from build123d import *

# Parameters (mm, degrees)
PAD050_DEPTH = 5
SKETCH054_R  = 10
PAD051_DEPTH = 5
SKETCH055_R  = 2.2
HOLE_DEPTH   = 25
SKETCH056_R  = 3
POCKET_DEPTH = 10.001


with BuildPart() as part:
    # Sketch053 → Pad050 (new body)
    with BuildSketch(Plane.XY):
        with BuildLine():
            Line((-21.5, 3.888093), (-21.5, -3.888093))
            Line((-21.5, -3.888093), (-6.644741, -10.57367))
            ThreePointArc((-6.644741, -10.57367), (0, -12), (6.644741, -10.57367))
            Line((6.644741, -10.57367), (21.5, -3.888093))
            Line((21.5, -3.888093), (21.5, 3.888093))
            Line((21.5, 3.888093), (6.644741, 10.57367))
            ThreePointArc((6.644741, 10.57367), (0, 12), (-6.644741, 10.57367))
            Line((-6.644741, 10.57367), (-21.5, 3.888093))
        make_face()
    extrude(amount=PAD050_DEPTH)

    # Sketch054 (on Face10 of Pad050) → Pad051 (join)
    with BuildSketch(Plane.XY.offset(5)):
        Circle(SKETCH054_R)
    extrude(amount=PAD051_DEPTH)

    # Sketch055 (on Face10 of Pad050) → Hole (cut)
    with BuildSketch(Plane.XY.offset(5)):
        with Locations((-16, 0)):
            Circle(SKETCH055_R)
        with Locations((16, 0)):
            Circle(SKETCH055_R)
    extrude(amount=-HOLE_DEPTH, mode=Mode.SUBTRACT)

    # Sketch056 (on Face14 of Hole) → Pocket (cut, through all)
    with BuildSketch(Plane.XY.offset(10)):
        Circle(SKETCH056_R)
    extrude(amount=-POCKET_DEPTH, mode=Mode.SUBTRACT)


solid = part.part
For this review, take the finished solid that the model builds, in its own axes (mm). A direction names the side the tool comes from. Coordinates: 2 decimals unless noted, no trailing zeros. Order: outer loops, then holes, each group sorted by start corner. A loop starts at its lowest first (then second) coordinate and runs counter-clockwise, first axis right, second up. Notation, with made-up numbers: (0.25, 89.5) - (49.25, 89.5) arc R16 ccw to (49.25, 106.5) - close; hole circle Ø10 at (87, -32.5). An arc over 180 degrees is marked (long way). Use one line per item in the form item = value.
Q1. For P1, Ø5, axis at x = -16, y = 0, coming from the +Z side; P2, Ø3, axis at x = -6.5, z = 7.5, coming from the -Y side; P3, Ø1, axis at x = -7.5, z = 5, coming from the +Y side; P4, Ø3.5, axis at x = 0, y = 0, coming from the +Z side, all flat-tipped, find the tip position at first contact; note any pin that passes through.
Checked values:
P1 = 5
P2 = -8.66
P3 = 10.41
P4 = through
Q2. Consider section A-A (z = 0.5). Give the boundary of the cut face in (x, y), then the cut area to 3 significant figures.
Checked values:
outline = (-21.5, -3.89) - (-6.64, -10.57) arc R16.19 ccw to (6.64, -10.57) - (21.5, -3.89) - (21.5, 3.89) - (6.64, 10.57) arc R16.19 ccw to (-6.64, 10.57) - (-21.5, 3.89) - close; hole circle Ø4.4 at (-16, 0); hole circle Ø6 at (0, 0); hole circle Ø4.4 at (16, 0)
area = 678 mm2
Q3. Consider section B-B (x = 0). Give the boundary of the cut face in (y, z).
Checked values:
outline = (-12, 0) - (-3, 0) - (-3, 10) - (-10, 10) - (-10, 5) - (-12, 5) - close; (3, 0) - (12, 0) - (12, 5) - (10, 5) - (10, 10) - (3, 10) - close
Q4. For faces 1 (the cylindrical face through (-2.17, -9.76, 7.46)), 2 (the cylindrical face through (-13.968, -0.843, 2.535)), list the 3-axis set-ups (+Z, -Z, +X, -X, +Y, -Y) from which the entire face can be reached by the end or side of a thin tool; tool diameter is ignored.
Checked values:
face_1 = +Z
face_2 = +Z, -Z
Q5. Draft analysis for pull direction X (two halves, no side actions). For faces 3 (the flat face through (21.5, 0, 2)), 4 (the cylindrical face through (-3, 0, 5)), 5 (the flat face through (-10, 3, 5)), state which applies: +X half, -X half, draft (parallel to the pull), parting line (faces both ways), or undercut.
Checked values:
face_3 = +X half
face_4 = undercut
face_5 = draft
Q6. Consider section C-C (y = 0). Give the boundary of the cut face in (x, z).
Checked values:
outline = (-21.5, 0) - (-18.2, 0) - (-18.2, 5) - (-21.5, 5) - close; (-13.8, 0) - (-3, 0) - (-3, 10) - (-10, 10) - (-10, 5) - (-13.8, 5) - close; (3, 0) - (13.8, 0) - (13.8, 5) - (10, 5) - (10, 10) - (3, 10) - close; (18.2, 0) - (21.5, 0) - (21.5, 5) - (18.2, 5) - close
Q7. For probe 1 along Y at (x, z) = (0, 8.25); probe 2 along Y at (x, z) = (0, 3.5); probe 3 along X at (y, z) = (-0.5, 4.5), list the stretches that pass through material, from the lowest coordinate up. Write a range as from..to.
Checked values:
probe_1 = -10..-3, 3..10
probe_2 = -12..-3, 3..12
probe_3 = -21.5..-18.14, -13.86..-2.96, 2.96..13.86, 18.14..21.5
Q8. Consider section D-D (y = 5.25). Give the boundary of the cut face in (x, z).
Checked values:
outline = (-18.47, 0) - (18.47, 0) - (18.47, 5) - (8.51, 5) - (8.51, 10) - (-8.51, 10) - (-8.51, 5) - (-18.47, 5) - close
